```python
from build123d import *

# Parameters (mm, degrees)
F6_DEPTH = 38.1


with BuildPart() as f2:
    # F0 (on Right) → F2 (revolve)
    with BuildSketch(Plane.YZ):
        Polygon((-35.56, 31.75), (0, 25.4), (0.5401693397, 28.5287657554), (-35.56, 34.975224566), align=None)
    revolve(axis=Axis((0, -17.78, 0), (0, -1, 0)))

    # F1 (on Top) → F3 (revolve)
    with BuildSketch(Plane.XY):
        with BuildLine():
            Line((25.4, 3.175), (25.4, 0))
            Line((25.4, 0), (28.575, 0))
            ThreePointArc((28.575, 0), (27.6450640303, 2.2450640303), (25.4, 3.175))
        make_face()
    revolve(axis=Axis((0, 1.5875, 0), (0, 1, 0)))

    # F0 (on Right) → F4 (revolve)
    with BuildSketch(Plane.YZ):
        Polygon((-43.18, 31.75), (-35.56, 31.75), (-35.56, 34.975224566), (-35.56, 38.1), (-43.18, 38.1), align=None)
    revolve(axis=Axis((0, -39.37, 0), (0, -1, 0)))

    # F5 (on Right) → F6 (cut)
    with BuildSketch(Plane.YZ):
        with BuildLine():
            Line((-35.5086600387, 10.16), (-35.5086600387, 0))
            Line((-35.5086600387, 0), (-35.5086600387, -10.16))
            Line((-35.5086600387, -10.16), (-25.3486600387, -10.16))
            ThreePointArc((-25.3486600387, -10.16), (-18.1644551419, -7.1842048969), (-15.1886600387, 0))
            ThreePointArc((-15.1886600387, 0), (-18.1644551419, 7.1842048969), (-25.3486600387, 10.16))
            Line((-25.3486600387, 10.16), (-35.5086600387, 10.16))
        make_face()
    extrude(amount=-F6_DEPTH, mode=Mode.SUBTRACT)


solid = f2.part
```
Input: part model. Units: mm. Frame: model coordinates. A direction names the side the tool comes from. Round coordinates to 2 decimals unless told otherwise and drop trailing zeros. Loops run counter-clockwise (first coordinate to the right, second up) from the corner with the lowest first, then second, coordinate; pieces in that order, holes last. Notation, with made-up numbers: M -25,-33 L -2,-33 A4 ccw -2,-29 Z; hole C 59,8 d9. An arc over 180 degrees is marked long. Answer in a Markdown table with one row per item. Add a question column.
1. Set-up query: faces 5 (the face through (-31, -43.18, -9)), 6 (the face through (-31, -30, 10.16)). Return all of +Z, -Z, +X, -X, +Y, -Y with unobstructed straight access to the full face (end or side cutting, diameter ignored); none if empty.
2. Ray query, probe 1 along X at (y, z) = (-38, 0); probe 2 along Y at (x, z) = (-17.5, 31.5); probe 3 along X at (y, z) = (-35, 29). Return the intervals inside material, ascending.
3. Section B-B (z = 1). Give the number of separate pieces and of enclosed holes in the cut face, and give its area (3 significant figures).
4. Section C-C (y = -28). Output: boundary loops of the cut face in (x, z), and give its area (3 significant figures).
5. Contact query for flat-ended pins moving along their axis: pin 1 (4 mm diameter, centred on x = -29.5, y = -18, fed in from +Z); pin 2 (1.5 mm diameter, centred on y = -23.5, z = -20.5, fed in from -X); pin 3 (10 mm diameter, centred on x = -11.5, y = -11.5, fed in from -Z). Output: stop coordinate, or through.
6. Mould query, pull axis Z, two halves, no side actions, for faces 1 (the face through (27.163, -13.58, -6.032)), 2 (the face through (30.34, -13.75, -6.74)), 3 (the face through (30.995, -39.317, -6.883)), 4 (the face through (31, -35.56, -17)). Classes: released by +Z, released by -Z, zero draft, split by the parting line, or undercut.
Values follow:
| question | item | result |
|---|---|---|
| 1 | face 5 | +Z, -Z, +X, -X, -Y |
| 1 | face 6 | -X |
| 2 | probe 1 | -38.1 to -31.75, 31.75 to 38.1 |
| 2 | probe 2 | -43.18 to -35.56 |
| 2 | probe 3 | -19.37 to -12.68, 12.68 to 19.37 |
| 3 | separate pieces | 3 |
| 3 | enclosed holes | 0 |
| 3 | area | 277 mm^2 |
| 4 | outline | M -32.05,-10.16 A33.63 ccw long -32.05,10.16 L -28.65,10.16 A30.4 cw long -28.65,-10.16 Z |
| 4 | area | 582 mm^2 |
| 5 | pin 1 | z = 16.12 |
| 5 | pin 2 | x = -26.24 |
| 5 | pin 3 | z = -30.3 |
| 6 | face 1 | undercut |
| 6 | face 2 | split by the parting line |
| 6 | face 3 | undercut |
| 6 | face 4 | zero draft |
